Geometry check sheet. Reference: the model listing, model coordinates, mm. A direction names the side the tool comes from. Give positions to 0.01 mm unless a question says otherwise; leave off trailing zeros. Write each loop counter-clockwise with the first axis right and the second up, starting at its lowest first coordinate (ties: lowest second). Pieces come first, ordered by that corner, then holes.
(1) Cross-section at B-B (z = -12.25). Record the boundary of the cut face in (x, y), and give its area (3 significant figures).
(2) Depth check by flat-ended pin: P1, Ø1.9, axis at x = 11.45, z = -11.59, coming from the +Y side; P2, Ø2, axis at y = 19, z = -3, coming from the +X side; P3, Ø3, axis at x = -2.5, y = 7, coming from the +Z side; P4, Ø10, axis at x = 0.5, y = 4.5, coming from the -Z side. Enter the tip coordinate at first touch or a pass-through.
(3) Mould release check, pull along X, two halves, no side actions. Record for faces 4 (the flat face through (7, 0, -7)), 5 (the flat face through (-0.148, 12, 3)), 6 (the cylindrical face through (12.44, 2.46, -12)): +X half, -X half, draft (parallel to the pull), parting line (faces both ways), or undercut.
(4) Cross-section at D-D (x = 17.5). Record the boundary of the cut face in (y, z), and give its area (3 significant figures).
(5) Tool access check on faces 1 (the flat face through (-3, 12, 0.006)), 2 (the flat face through (1, 23.9, 0.1)), 3 (the flat face through (2.317, 15.332, -2.529)). Record the directions out of +Z, -Z, +X, -X, +Y, -Y that give a thin tool (end or side, any length) a straight path to the whole face; none if there is none.
(6) Thickness scan on line 1 along Z through (x, y) = (0.5, 16.25); line 2 along Z through (x, y) = (3, 4); line 3 along X through (y, z) = (8.5, -4.75). Record the ranges inside material, lowest first.
(7) Cross-section at A-A (x = 15). Record the boundary of the cut face in (y, z), and give its area (3 significant figures).
(8) Cross-section at C-C (y = 7.5). Record the boundary of the cut face in (x, z), and give its area (3 significant figures).
Autodesk Inventor part; units mm, degrees
ref_plane "YZ Plane" through (0, 0, 0) normal (1, 0, 0) x (0, 1, 0)
ref_plane "XZ Plane" through (0, 0, 0) normal (0, 1, 0) x (-1, 0, 0)
ref_plane "XY Plane" through (0, 0, 0) normal (0, 0, 1) x (1, 0, 0)
sketch "Sketch1" plane through (0, 0, 0) normal (0, 1, 0) x (-1, 0, 0)
  arc A0 (-0.158902, 2.527129) -> (-1.647898, 1.801809) centre (0.148153, 0.005757) ccw
  arc A1 (-0.158902, 2.527129) -> (-1.647898, 1.801809) centre (0.148153, 0.005757) ccw
  arc A2 (1.944204, -1.790294) -> (2.669525, -0.301298) centre (0.148153, 0.005757) ccw
  arc A3 (1.944204, -1.790294) -> (2.669525, -0.301298) centre (0.148153, 0.005757) ccw
  arc A4 (0.148153, 2.545757) -> (-1.647898, 1.801809) centre (0.148153, 0.005757) ccw
  line L0 (0.148153, 5.005757) -> (0.148153, 2.545757)
  line L1 (0.148153, 0.005757) -> (2.688153, 0.005757)
  line L2 (-1.647898, 1.801809) -> (-4.147898, -0.698191)
  arc A5 (1.944204, -1.790294) -> (2.688153, 0.005757) centre (0.148153, 0.005757) ccw
  line L3 (-4.147898, -0.698191) -> (-4.851847, 0.005757)
  arc A6 (0.148153, 2.545757) -> (-1.647898, 1.801809) centre (0.148153, 0.005757) ccw
  arc A7 (0.148153, 2.545757) -> (-1.647898, 1.801809) centre (0.148153, 0.005757) ccw
  arc A8 (-0.158902, 2.527129) -> (-1.647898, 1.801809) centre (0.148153, 0.005757) ccw
  arc A9 (-0.158902, 2.527129) -> (-1.647898, 1.801809) centre (0.148153, 0.005757) ccw
  line L4 (-4.851847, 0.005757) -> (0.148153, 5.005757)
  line L5 (-4.851847, 0.005757) -> (0.148153, 5.005757)
  line L6 (0.148153, 5.005757) -> (0.148153, 2.545757)
  arc A10 (0.148153, 2.545757) -> (-1.647898, 1.801809) centre (0.148153, 0.005757) ccw
  line L7 (-1.647898, 1.801809) -> (-4.147898, -0.698191)
  line L8 (-4.147898, -0.698191) -> (-4.851847, 0.005757)
  arc A11 (1.944204, -1.790294) -> (2.688153, 0.005757) centre (0.148153, 0.005757) ccw
  arc A12 (1.944204, -1.790294) -> (2.669525, -0.301298) centre (0.148153, 0.005757) ccw
  arc A13 (1.944204, -1.790294) -> (2.669525, -0.301298) centre (0.148153, 0.005757) ccw
  arc A14 (1.944204, -1.790294) -> (2.688153, 0.005757) centre (0.148153, 0.005757) ccw
  line L9 (-4.147898, -0.698191) -> (-0.555796, -4.290294)
  line L10 (0.148153, 1.005757) -> (0.148153, 0.005757)
  line L11 (0.148153, 1.005757) -> (0.148153, 0.005757)
  line L12 (0.148153, 2.545757) -> (0.148153, 0.005757)
  line L13 (0.148153, 5.005757) -> (0.148153, 2.545757)
  line L14 (0.148153, 5.005757) -> (0.148153, 1.005757)
  line L15 (0.148153, 0.005757) -> (1.148153, 0.005757)
  line L16 (1.148153, 0.005757) -> (5.148153, 0.005757)
  line L17 (2.688153, 0.005757) -> (5.148153, 0.005757)
  line L18 (0.148153, 0.005757) -> (2.688153, 0.005757)
  line L19 (5.148153, 0.005757) -> (0.148153, -4.994243)
  line L20 (0.148153, -4.994243) -> (5.148153, 0.005757)
  line L21 (-4.147898, -0.698191) -> (-4.851847, 0.005757)
  line L22 (-4.147898, -0.698191) -> (-0.555796, -4.290294)
  line L23 (0.148153, -4.994243) -> (-0.555796, -4.290294)
  line L24 (-4.851847, 0.005757) -> (0.148153, -4.994243)
  line L25 (-4.851847, 0.005757) -> (0.148153, -4.994243)
  line L26 (0.148153, 5.005757) -> (-4.851847, 0.005757)
  line L27 (-4.851847, 0.005757) -> (0.148153, 5.005757)
  line L28 (0.148153, 5.005757) -> (-4.851847, 0.005757)
  line L29 (0.148153, -4.994243) -> (-0.555796, -4.290294)
  arc A15 (1.944204, -1.790294) -> (2.688153, 0.005757) centre (0.148153, 0.005757) ccw
  line L30 (-0.555796, -4.290294) -> (1.944204, -1.790294)
  line L31 (2.688153, 0.005757) -> (5.148153, 0.005757)
  line L32 (5.148153, 0.005757) -> (0.148153, -4.994243)
  line L33 (0.148153, -4.994243) -> (-0.555796, -4.290294)
  line L34 (-0.555796, -4.290294) -> (1.944204, -1.790294)
  arc A16 (1.944204, -1.790294) -> (2.688153, 0.005757) centre (0.148153, 0.005757) ccw
  line L35 (2.688153, 0.005757) -> (5.148153, 0.005757)
  line L36 (5.148153, 0.005757) -> (0.148153, -4.994243)
  arc A17 (0.148153, 2.545757) -> (-1.647898, 1.801809) centre (0.148153, 0.005757) ccw
  circle A18 centre (-2.355005, -2.497401) radius 1.5
  circle A19 centre (-2.355005, -2.497401) radius 1.5
  circle A20 centre (-2.355005, -2.497401) radius 1.5
  circle A21 centre (-2.355005, -2.497401) radius 1.5
  circle A22 centre (-2.355005, -2.497401) radius 1.5
  line L37 (0.148153, 5.005757) -> (0.148153, 1.005757)
  arc A23 (0.148153, 1.005757) -> (1.148153, 0.005757) centre (0.148153, 0.005757) ccw
  line L38 (0.148153, -4.994243) -> (5.148153, 0.005757)
  line L39 (1.148153, 0.005757) -> (5.148153, 0.005757)
  line L40 (0.148153, 0.005757) -> (1.148153, 0.005757)
  arc A24 (0.148153, 1.005757) -> (1.148153, 0.005757) centre (0.148153, 0.005757) ccw
  line L41 (0.148153, 0.005757) -> (1.148153, 0.005757)
  line L42 (0.148153, 1.005757) -> (0.148153, 0.005757)
  arc A25 (0.148153, 1.005757) -> (1.148153, 0.005757) centre (0.148153, 0.005757) ccw
  arc A26 (0.148153, 1.005757) -> (1.148153, 0.005757) centre (0.148153, 0.005757) ccw
  arc A27 (0.148153, 1.005757) -> (1.148153, 0.005757) centre (0.148153, 0.005757) ccw
  line L43 (0.148153, 5.005757) -> (-4.851847, 0.005757)
  line L44 (-4.851847, 0.005757) -> (0.148153, -4.994243)
  line L45 (0.148153, -4.994243) -> (5.148153, 0.005757)
  line L46 (1.148153, 0.005757) -> (5.148153, 0.005757)
  arc A28 (0.148153, 1.005757) -> (1.148153, 0.005757) centre (0.148153, 0.005757) ccw
  line L47 (0.148153, 5.005757) -> (0.148153, 1.005757)
  line L48 (0.148153, 2.545757) -> (0.148153, 0.005757)
  arc A29 (-1.647898, 1.801809) -> (1.944204, -1.790294) centre (0.148153, 0.005757) ccw
  circle A30 centre (0.148153, 0.005757) radius 2.54
  line L49 (0.148153, -3.586345) -> (-3.443949, 0.005757)
  line L50 (-1.647898, -1.790294) -> (-2.355005, -2.497401)
  circle A31 centre (-2.355005, -2.497401) radius 2.54
  point P0 (0, 0)
  point P1 (1.148153, 0.005757)
extrude "Extrusion1" add sketch "Sketch1" along normal blind 23.9 contours A4 L12 A23 A31 A29 A0 | A0 L2 L3 L4 L0 A4 | A29 A31 L49 L2 | L49 A31 L2 | A31 A29 A18 | A29 A18 L49 A31 | A5 A2 A29 A31 A23 L1 | L16 L19 L23 L30 A2 A5 | A31 L49 A18 L9 | A29 L49 A18 | A18 A29 | A18 L49 L50 L9 | A31 L49 L30 | L9 A18 L49 A31 | A29 A31 L49 A18 | A18 L49 A29 | L49 A18 L9 L50 | L30 L49 A31 A29
sketch "Sketch2" plane through (0, 0, 0) normal (0, -1, 0) x (1, 0, 0)
  line L0 (4.851847, 0.005757) -> (-0.148153, -4.994243)
  line L1 (2.351847, -2.494243) -> (17.908196, -18.050592)
  circle A0 centre (11.448069, -11.590464) radius 1.075
  circle A1 centre (15.690709, -15.833105) radius 1.075
  line L2 (-0.148153, 1.005757) -> (-0.148153, 5.005757)
  line L3 (-0.148153, 5.005757) -> (4.851847, 0.005757)
  line L4 (-0.148153, 5.005757) -> (4.851847, 0.005757)
  line L5 (-0.148153, -4.994243) -> (-5.148153, 0.005757)
  line L6 (-5.148153, 0.005757) -> (-0.148153, -4.994243)
  line L7 (2.351847, -2.494243) -> (4.119614, -0.726476)
  line L8 (4.119614, -0.726476) -> (0.58408, -4.26201)
  line L9 (0.58408, -4.26201) -> (16.044263, -19.722192)
  line L10 (4.119614, -0.726476) -> (19.579797, -16.186658)
  line L11 (17.908196, -18.050592) -> (17.81203, -18.146758)
  line L12 (17.81203, -18.146758) -> (16.140429, -19.818359)
  line L13 (16.140429, -19.818359) -> (16.044263, -19.722192)
  line L14 (17.908196, -18.050592) -> (19.675963, -16.282825)
  line L15 (19.675963, -16.282825) -> (19.579797, -16.186658)
  point P0 (0, 0)
  dimension "d2" = 22
  dimension "d5" = 2.15
  dimension "d6" = 2.15
  dimension "d7" = 2.5
  dimension "d8" = 5
extrude "Extrusion2" add sketch "Sketch2" against normal blind 5 contours L10 L15 L14 L1 A1 A0 L0 | L1 A0 A1 L11 L12 L13 L9 L0
fillet "Fillet1" radius 2 2 edges at (4.1196, 2.5, -0.7265) (0.5841, 2.5, -4.262)
fillet "Fillet2" radius 2 1 edges at (2.3518, 5, -2.4942)
sketch "Sketch3" plane through (0, 5, 0) normal (0, 1, 0) x (1, 0, 0)
  circle A0 centre (11.448069, 11.590464) radius 1.075
  circle A1 centre (15.690709, 15.833105) radius 1.075
  point P0 (0, 0)
properties part number "ALUMFINGER_3DPrint"
Reply:
1. outline: (8.57, 0) - (10.6, 0) - (10.6, 5) - (8.57, 5) - close; (12.3, 0) - (15.64, 0) - (15.64, 5) - (12.3, 5) - close
1. area: 26.9 mm2
2. P1: passes through
2. P2: stops at x = 2.85
2. P3: stops at z = 0.01
2. P4: stops at z = -9.18
3. face 4: draft
3. face 5: -X half
3. face 6: undercut
4. outline: (0, -18.46) - (5, -18.46) - (5, -14.11) - (0, -14.11) - close
4. area: 21.8 mm2
5. face 1: +Z, -X, +Y, -Y
5. face 2: +Z, -Z, +X, -X, +Y
5. face 3: -Z, +X, +Y
6. line 1: z = -4.35 to -0.76, 0.77 to 4.36
6. line 2: z = -6.68 to 1.86
6. line 3: x = -0.39 to 0.1
7. outline: (0, -18.68) - (5, -18.68) - (5, -16.66) - (0, -16.66) - close; (0, -15.01) - (5, -15.01) - (5, -11.61) - (0, -11.61) - close
7. area: 27.1 mm2
8. outline: (-5.15, 0.01) - (-0.15, -4.99) - (4.85, 0.01) - (-0.15, 5.01) - (-0.15, 1.01) arc R1 cw (long way) to (-1.15, 0.01) - close
8. area: 35.1 mm2
